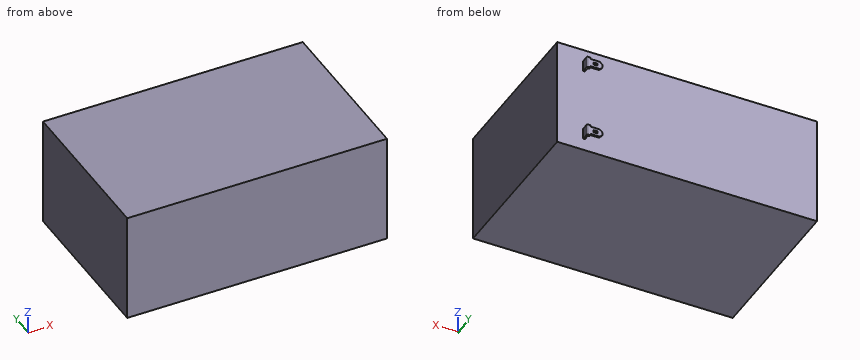
from build123d import *

# Parameters (mm, degrees)
SKETCH1_W           = 150
SKETCH1_H           = 63.5
BOSS_EXTRUDE1_DEPTH = 94.2
SKETCH3_W           = 2.3
SKETCH3_H           = 1.4
BOSS_EXTRUDE2_DEPTH = 4.4
SKETCH4_W           = 6.8
SKETCH4_H           = 3.4
CUT_EXTRUDE1_DEPTH  = 189.186636082


with BuildPart() as part:
    # Sketch1 → Boss-Extrude1 (new body)
    with BuildSketch(Plane(origin=(0, 0, 0), x_dir=(1, 0, 0), z_dir=(0, 1, 0))):
        with Locations((75, 31.75)):
            Rectangle(SKETCH1_W, SKETCH1_H)
    extrude(amount=BOSS_EXTRUDE1_DEPTH)

    # Sketch3 → Boss-Extrude2 (add)
    with BuildSketch(Plane(origin=(0, 94.2, 0), x_dir=(1, 0, 0), z_dir=(0, 1, 0))):
        Polygon((135, 7), (135, 13.4), (133, 13.4), (133, 12.5), (127.6, 12.5), (126.2, 11.1), (126.2, 9.3), (127.6, 7.9), (133, 7.9), (133, 7), align=None)
        with Locations((130.15, 10.2)):
            Rectangle(SKETCH3_W, SKETCH3_H, mode=Mode.SUBTRACT)
    boss_extrude2 = extrude(amount=BOSS_EXTRUDE2_DEPTH)

    # Sketch4 → Cut-Extrude1 (cut, through all)
    with BuildSketch(Plane.XY.offset(-7)):
        with Locations((129.6, 95.9)):
            Rectangle(SKETCH4_W, SKETCH4_H)
        with BuildLine():
            Line((133, 94.2), (134, 94.2))
            Line((134, 94.2), (134, 97.1))
            ThreePointArc((134, 97.1), (133.853553391, 97.453553391), (133.5, 97.6))
            Line((133.5, 97.6), (133, 97.6))
            Line((133, 97.6), (133, 94.2))
        make_face()
        with BuildLine():
            ThreePointArc((134.5, 98.6), (134.853553391, 98.453553391), (135, 98.1))
            Line((135, 98.1), (135, 98.6))
            Line((135, 98.6), (134.5, 98.6))
        make_face()
    cut_extrude1 = extrude(amount=-CUT_EXTRUDE1_DEPTH, mode=Mode.SUBTRACT)

    # Mirror1: Boss-Extrude2, Cut-Extrude1 across plane
    add(boss_extrude2.mirror(Plane.XY.offset(-31.75)))
    add(cut_extrude1.mirror(Plane.XY.offset(-31.75)), mode=Mode.SUBTRACT)


solid = part.part
CAD build for the part. Positions are in the model's coordinates, mm. Coordinates: 2 decimals unless noted, no trailing zeros. Loops run counter-clockwise (first coordinate to the right, second up) from the corner with the lowest first, then second, coordinate; pieces in that order, holes last. Notation, with made-up numbers: (-17.5, -24) - (-11.5, -24) arc R21 ccw to (-11.5, 6) - close; hole circle Ø11 at (21, 20.5). An arc over 180 degrees is marked (long way). Write item = value, one per line. Start each with the question number.
Q1. Flat gauge pins, fed straight in: pin 1 Ø2 at (x, z) = (133, -39.5) entering from +Y; pin 2 Ø1.1 at (x, y) = (130, 98) entering from +Z; pin 3 Ø1.1 at (y, z) = (98.5, -53) entering from -X. Where does each tip first touch, or does it go through?
Q2. Drill centre line: L1, parallel to Y at x = 78.5, z = -43. Where is it in solid material? Low to high.
Q3. Cut at B-B, the plane z = -3.5. List the corners of the cut face in (x, y).
Q4. Cut at A-A, the plane x = 15.5. List the corners of the cut face in (y, z).
Computed:
q1.pin_1 = 94.2
q1.pin_2 = -7.9
q1.pin_3 = 126.2
q2.L1 = 0 to 94.2
q3.outline = (0, 0) - (150, 0) - (150, 94.2) - (0, 94.2) - close
q4.outline = (0, -63.5) - (94.2, -63.5) - (94.2, 0) - (0, 0) - close
